Can you work these out from the model? Positions are in its coordinate system, mm. A direction names the side the tool comes from. Round coordinates to 2 decimals unless told otherwise and drop trailing zeros. Order: outer loops, then holes, each group sorted by start corner. A loop starts at its lowest first (then second) coordinate and runs counter-clockwise, first axis right, second up. Notation, with made-up numbers: (-2.5, 55) -> (54.5, 55) arc R12 ccw to (54.5, 78) -> close; hole circle Ø2 at (14, 69). An arc over 180 degrees is marked (long way). Use a Markdown table: item, result. Add a question column.
Q1. I need wall thicknesses on line 1 along X through (y, z) = (17.75, 0); line 2 along Y through (x, z) = (-30.5, 24); line 3 along X through (y, z) = (6.25, 17.5). Which ranges of each line are inside material? Lowest first, please. Write a range as [from, to].
Q2. I'm going to push flat-ended pins straight in: pin 1 Ø8 at (y, z) = (13.5, -19.5) entering from +X; pin 2 Ø1 at (x, z) = (-32, 8.5) entering from +Y; pin 3 Ø1 at (y, z) = (12, 22) entering from +X; pin 4 Ø19 at (x, z) = (-2.5, -2.5) entering from -Y. Where does each tip first touch, or does it pass through?
Q3. For faces 1 (the face through (-6.64, 19.37, -29.9)), 2 (the face through (2, 10, 6)), which set-ups out of +Z, -Z, +X, -X, +Y, -Y let a thin tool reach every point of the face, with its end or its side?
Q4. If we section it at B-B on y = 7: List the corners of the cut face in (x, z) for me.
Q5. We'd pull the mould along Z, two halves only. Please class faces 3 (the face through (7.535, 4.93, -4.27)), 4 (the face through (7.465, 4.93, 4.391)), 5 (the face through (-0.42, 20, 6.25)), 6 (the face through (-8.67, 5.07, 39.05)): +Z half, -Z half, draft (parallel to the pull), parting line (faces both ways), or undercut.
Q6. If we section it at A-A on x = 0: List the corners of the cut face in (y, z) for me, plus the area to 3 significant figures.
Autodesk Inventor part; units mm, degrees
sketch "Esboço1" plane through (0, 0, 0) normal (0, 0, 1) x (1, 0, 0)
  line L0 (-40, 0) -> (-40, 10)
  line L1 (-40, 10) -> (-30, 20)
  line L2 (-30, 20) -> (0, 20)
  line L3 (-40, 0) -> (0, 0)
  line L4 (0, 20) -> (0, 0)
  line L5 (0, -4) -> (0, 24)
  dimension "d0" = 40
  dimension "d1" = 10
  dimension "d6" = 135
  dimension "d7" = 30
revolve "Revolução1" add sketch "Esboço1" angle 360 mid plane about axis through (0, -10, 0) along (0, 1, 0)
sketch "Esboço2" plane through (0, 20, 0) normal (0, 1, 0) x (1, 0, 0)
  circle A0 centre (0, 0) radius 6.1
  dimension "d9" = 12.2
extrude "Extrusão1" cut sketch "Esboço2" against normal through all
sketch "Esboço3" plane through (0, 0, 0) normal (0, -1, 0) x (1, 0, 0)
  line L0 (5, 8.6603) -> (10, 0)
  line L1 (10, 0) -> (5, -8.6603)
  line L2 (5, -8.6603) -> (-5, -8.6603)
  line L3 (-5, -8.6603) -> (-10, 0)
  line L4 (-10, 0) -> (-5, 8.6603)
  line L5 (-5, 8.6603) -> (5, 8.6603)
  point P0 (0, 0)
  point P1 (0, 0)
  point P2 (0, 8.6603)
  dimension "d12" = 10
extrude "Extrusão2" cut sketch "Esboço3" against normal blind 10
properties part number "Sessao9__08_04_2025_0001_001" material "Ouro"
Answer below:
| question | item | result |
|---|---|---|
| 1 | line 1 | [-32.25, -6.1], [6.1, 32.25] |
| 1 | line 2 | [0, 11.19] |
| 1 | line 3 | [-35.97, 35.97] |
| 2 | pin 1 | x = 35.94 |
| 2 | pin 2 | y = 17.39 |
| 2 | pin 3 | x = 31.69 |
| 2 | pin 4 | y = 0 |
| 3 | face 1 | +Y |
| 3 | face 2 | -Y |
| 4 | outline | circle Ø80 at (0, 0); hole (-10, 0) -> (-5, -8.66) -> (5, -8.66) -> (10, 0) -> (5, 8.66) -> (-5, 8.66) -> close |
| 5 | face 3 | undercut |
| 5 | face 4 | undercut |
| 5 | face 5 | draft |
| 5 | face 6 | parting line |
| 6 | outline | (0, -40) -> (10, -40) -> (20, -30) -> (20, -6.1) -> (10, -6.1) -> (10, -8.66) -> (0, -8.66) -> close; (0, 8.66) -> (10, 8.66) -> (10, 6.1) -> (20, 6.1) -> (20, 30) -> (10, 40) -> (0, 40) -> close |
| 6 | area | 1,200 mm² |
